```python
from build123d import *

# Parameters (mm, degrees)
ESQUISSE1_W             = 330
ESQUISSE1_H             = 180
BOSS_EXTRU_1_DEPTH      = 6
ESQUISSE2_W             = 60
ESQUISSE2_H             = 6
ESQUISSE2_W_2           = 134
ESQUISSE2_W_3           = 6
ESQUISSE2_H_2           = 40
ESQUISSE2_W_4           = 86
ESQUISSE2_W_5           = 80
ENL_V_MAT_ENCOCHE_DEPTH = 376.946804748


with BuildPart() as part:
    # Esquisse1 → Boss.-Extru.1 (new body)
    with BuildSketch(Plane.XY):
        with Locations((-165, 90)):
            Rectangle(ESQUISSE1_W, ESQUISSE1_H)
    extrude(amount=BOSS_EXTRU_1_DEPTH)

    # Esquisse2 → Enlèv. mat encoche (cut, through all)
    with BuildSketch(Plane.XY.offset(6)):
        with Locations((-300, 177)):
            Rectangle(ESQUISSE2_W, ESQUISSE2_H)
        with Locations((-165, 177)):
            Rectangle(ESQUISSE2_W_2, ESQUISSE2_H)
        with Locations((-30, 177)):
            Rectangle(ESQUISSE2_W, ESQUISSE2_H)
        with Locations((-327, 123)):
            Rectangle(ESQUISSE2_W_3, ESQUISSE2_H_2)
        with Locations((-327, 57)):
            Rectangle(ESQUISSE2_W_3, ESQUISSE2_H_2)
        with Locations((-3, 123)):
            Rectangle(ESQUISSE2_W_3, ESQUISSE2_H_2)
        with Locations((-3, 57)):
            Rectangle(ESQUISSE2_W_3, ESQUISSE2_H_2)
        with Locations((-287, 3)):
            Rectangle(ESQUISSE2_W_4, ESQUISSE2_H)
        with Locations((-165, 3)):
            Rectangle(ESQUISSE2_W_5, ESQUISSE2_H)
        with Locations((-43, 3)):
            Rectangle(ESQUISSE2_W_4, ESQUISSE2_H)
    extrude(amount=-ENL_V_MAT_ENCOCHE_DEPTH, mode=Mode.SUBTRACT)


solid = part.part
```
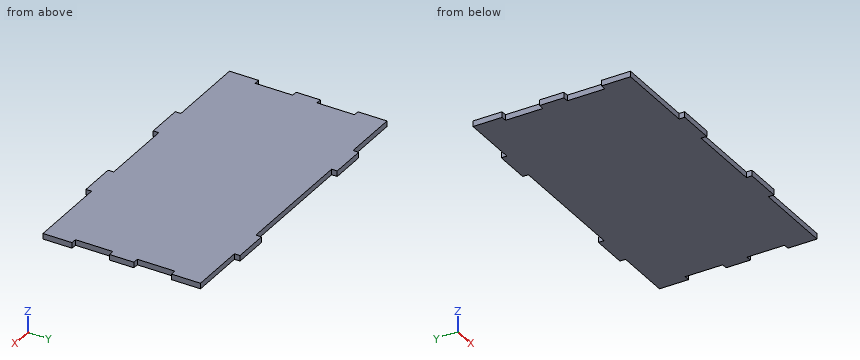
Can you work these out from the model? Positions are in its coordinate system, mm. Coordinates: 2 decimals unless noted, no trailing zeros. Write each loop counter-clockwise with the first axis right and the second up, starting at its lowest first coordinate (ties: lowest second). Pieces come first, ordered by that corner, then holes. Notation, with made-up numbers: M 6.25,-1 L 32.25,-1 A37 cw 32.25,36 Z; hole C 42,12 d1. An arc over 180 degrees is marked long. Write item = value, one per line. Start each with the question number.
Q1. I'm going to push flat-ended pins straight in: pin 1 (3 mm diameter, centred on y = 117.5, z = 3.5, fed in from -X); pin 2 (3 mm diameter, centred on y = 1.5, z = 2, fed in from +X); pin 3 (3 mm diameter, centred on x = -327, z = 4, fed in from +Y). Where does each tip first touch, or does it pass through?
Q2. If we section it at A-A, the plane y = 46: Write out the boundary of the cut face in (x, z).
Q3. If we section it at B-B, the plane x = -188: Write out the boundary of the cut face in (y, z), then the cut area to 3 significant figures.
Q4. If I drill on L1, parallel to Y at x = -216.5, z = 3.65; L2, parallel to Y at x = -296, z = 3.25; L3, parallel to X at y = 116.5, z = 0.4, over which ranges is the centre line in solid material (lowest first)? Write a range as [from, to].
Check sheet entries:
q1.pin_1 = -324
q1.pin_2 = -86
q1.pin_3 = 174
q2.outline = M -324,0 L -6,0 L -6,6 L -324,6 Z
q3.outline = M 6,0 L 174,0 L 174,6 L 6,6 Z
q3.area = 1,010 mm²
q4.L1 = [0, 174]
q4.L2 = [6, 174]
q4.L3 = [-324, -6]
